For this review, take the finished solid that the model builds, in its own axes (mm). A direction names the side the tool comes from. Round coordinates to 2 decimals unless told otherwise and drop trailing zeros. Loops run counter-clockwise (first coordinate to the right, second up) from the corner with the lowest first, then second, coordinate; pieces in that order, holes last. Notation, with made-up numbers: (-24.75, 1.5) -> (-11.75, 1.5) arc R20 ccw to (-11.75, 11.5) -> close; hole circle Ø6 at (7, 85). An arc over 180 degrees is marked (long way). One line per question, with ' | ' between items. Start each with the question number.
1. Consider section C-C (y = 77). Write out the cut boundary in (x, z) (3 decimals).
2. Draft analysis for pull direction X (two halves, no side actions). For faces 1 (the face through (-5.26, 22.01, 9.51)), 2 (the face through (10, 40, 0)), 3 (the face through (0, 40, 10)), state which applies: pulls with the +X half, pulls with the -X half, needs draft (parallel to the pull), parting line crosses it, or undercut.
3. Consider section D-D (y = 16.5). Write out the cut boundary in (x, z).
4. For faces 4 (the face through (0, 40, 9)), 5 (the face through (4.561, 60.023, 9.507)), list the 3-axis set-ups (+Z, -Z, +X, -X, +Y, -Y) from which the entire face can be reached by the end or side of a thin tool; tool diameter is ignored.
5. Consider section A-A (z = 4.75). Write out the cut boundary in (x, y).
6. Wall thickness on line 1 along Y through (x, z) = (-5, -9.65) (3 decimals); line 2 along X through (y, z) = (29.5, -1.5): over which ranges is each line inside the solid? List them lowest first.
7. For pin 1 Ø5 at (x, z) = (1.5, -7) entering from +Y, flat-tipped, find the tip position at first contact; note if it passes through.
8. Consider section B-B (x = 8.25). Write out the cut boundary in (y, z), and give its area (3 significant figures).
```python
from build123d import *

# Parameters (mm, degrees)
SKETCH_1_W          = 20
SKETCH_1_H          = 20
SKETCH_1_W_2        = 18
SKETCH_1_H_2        = 18
EXTRUDE_1_DEPTH     = 82
SKETCH_2_R          = 2.025
CUT_EXTRUDE_1_DEPTH = 21


with BuildPart() as part:
    # 草图1 → 凸台-拉伸1 (new body)
    with BuildSketch(Plane(origin=(0, 0, 0), x_dir=(1, 0, 0), z_dir=(0, 1, 0))):
        Rectangle(SKETCH_1_W, SKETCH_1_H)
        Rectangle(SKETCH_1_W_2, SKETCH_1_H_2, mode=Mode.SUBTRACT)
    extrude(amount=EXTRUDE_1_DEPTH)

    # 草图2 → 切除-拉伸1 (cut, through all)
    with BuildSketch(Plane.XY.offset(10)):
        with Locations((-5, 5)):
            Circle(SKETCH_2_R)
        with Locations((-5, 20)):
            Circle(SKETCH_2_R)
        with Locations((5, 20)):
            Circle(SKETCH_2_R)
        with Locations((5, 5)):
            Circle(SKETCH_2_R)
        with Locations((5, 77)):
            Circle(SKETCH_2_R)
        with Locations((-5, 77)):
            Circle(SKETCH_2_R)
        with Locations((-5, 62)):
            Circle(SKETCH_2_R)
        with Locations((5, 62)):
            Circle(SKETCH_2_R)
    extrude(amount=-CUT_EXTRUDE_1_DEPTH, mode=Mode.SUBTRACT)


solid = part.part
```
Answer block:
1) outline: (-10, -10) -> (-7.025, -10) -> (-7.025, -9) -> (-9, -9) -> (-9, 9) -> (-7.025, 9) -> (-7.025, 10) -> (-10, 10) -> close; (-2.975, -10) -> (2.975, -10) -> (2.975, -9) -> (-2.975, -9) -> close; (-2.975, 9) -> (2.975, 9) -> (2.975, 10) -> (-2.975, 10) -> close; (7.025, -10) -> (10, -10) -> (10, 10) -> (7.025, 10) -> (7.025, 9) -> (9, 9) -> (9, -9) -> (7.025, -9) -> close
2) face 1: undercut | face 2: pulls with the +X half | face 3: needs draft
3) outline: (-10, -10) -> (10, -10) -> (10, 10) -> (-10, 10) -> close; hole (-9, -9) -> (9, -9) -> (9, 9) -> (-9, 9) -> close
4) face 4: +Y, -Y | face 5: +Z, -Z
5) outline: (-10, 0) -> (-9, 0) -> (-9, 82) -> (-10, 82) -> close; (9, 0) -> (10, 0) -> (10, 82) -> (9, 82) -> close
6) line 1: y = 0 to 2.975, 7.025 to 17.975, 22.025 to 59.975, 64.025 to 74.975, 79.025 to 82 | line 2: x = -10 to -9, 9 to 10
7) pin 1: stops at y = 82
8) outline: (0, -10) -> (82, -10) -> (82, -9) -> (0, -9) -> close; (0, 9) -> (82, 9) -> (82, 10) -> (0, 10) -> close | area: 164 mm2
